```python
from build123d import *

# Parameters (mm, degrees)
SKETCH1_R           = 55
SKETCH1_R_2         = 3
BOSS_EXTRUDE1_DEPTH = 20
SKETCH2_R           = 52
CUT_EXTRUDE1_DEPTH  = 10
SKETCH3_R           = 73.645142789
CUT_EXTRUDE2_DEPTH  = 40
CUT_EXTRUDE4_START  = -58
CUT_EXTRUDE4_DEPTH  = 58
SKETCH5_R           = 2.5
CUT_EXTRUDE3_DEPTH  = 110


with BuildPart() as part:
    # Sketch1 → Boss-Extrude1 (new body)
    with BuildSketch(Plane.XY):
        Circle(SKETCH1_R)
        Circle(SKETCH1_R_2, mode=Mode.SUBTRACT)
    extrude(amount=BOSS_EXTRUDE1_DEPTH)

    # Sketch2 → Cut-Extrude1 (cut)
    with BuildSketch(Plane.XY.offset(20)):
        Circle(SKETCH2_R)
        with BuildLine():
            Line((-41.361950208, 16.620711788), (-41.361950208, -16.620711788))
            ThreePointArc((-41.361950208, -16.620711788), (0, -44.576439802), (41.361950208, -16.620711788))
            Line((41.361950208, -16.620711788), (41.361950208, 16.620711788))
            ThreePointArc((41.361950208, 16.620711788), (0, 44.576439802), (-41.361950208, 16.620711788))
        make_face(mode=Mode.SUBTRACT)
    extrude(amount=-CUT_EXTRUDE1_DEPTH, mode=Mode.SUBTRACT)

    # Sketch3 → Cut-Extrude2 (cut)
    with BuildSketch(Plane.XY.offset(20)):
        Circle(SKETCH3_R)
        with BuildLine():
            Line((-41.361950208, 16.620711788), (-41.361950208, -16.620711788))
            ThreePointArc((-41.361950208, -16.620711788), (0, -44.576439802), (41.361950208, -16.620711788))
            Line((41.361950208, -16.620711788), (41.361950208, 16.620711788))
            ThreePointArc((41.361950208, 16.620711788), (0, 44.576439802), (-41.361950208, 16.620711788))
        make_face(mode=Mode.SUBTRACT)
    extrude(amount=-CUT_EXTRUDE2_DEPTH, mode=Mode.SUBTRACT)

    # Sketch6 → Cut-Extrude4 (cut)
    with BuildSketch(Plane(origin=(0, 0, 0), x_dir=(-1, 0, 0), z_dir=(0, 0, -1)).offset(CUT_EXTRUDE4_START)):
        with BuildLine():
            ThreePointArc((-41.361950208, 16.620711788), (-37.775123844, 23.66641088), (-33, 29.967632295))
            Line((-33, 29.967632295), (-58.675122088, 18.005162572))
            Line((-58.675122088, 18.005162572), (-58.675122088, -19.387832384))
            Line((-58.675122088, -19.387832384), (-33, -29.967632295))
            ThreePointArc((-33, -29.967632295), (-37.775123844, -23.66641088), (-41.361950208, -16.620711788))
            Line((-41.361950208, -16.620711788), (-41.361950208, 16.620711788))
        make_face()
        with BuildLine():
            Line((-33, -29.967632295), (-33, 29.967632295))
            ThreePointArc((-33, 29.967632295), (-37.775123844, 23.66641088), (-41.361950208, 16.620711788))
            Line((-41.361950208, 16.620711788), (-41.361950208, -16.620711788))
            ThreePointArc((-41.361950208, -16.620711788), (-37.775123844, -23.66641088), (-33, -29.967632295))
        make_face()
        with BuildLine():
            Line((59.4434713, 26.815208095), (33, 29.967632295))
            ThreePointArc((33, 29.967632295), (37.775123844, 23.66641088), (41.361950208, 16.620711788))
            Line((41.361950208, 16.620711788), (41.361950208, -16.620711788))
            ThreePointArc((41.361950208, -16.620711788), (37.775123844, -23.66641088), (33, -29.967632295))
            Line((33, -29.967632295), (59.4434713, -14.291474717))
            Line((59.4434713, -14.291474717), (59.4434713, 26.815208095))
        make_face()
        with BuildLine():
            ThreePointArc((41.361950208, 16.620711788), (37.775123844, 23.66641088), (33, 29.967632295))
            Line((33, 29.967632295), (33, -29.967632295))
            ThreePointArc((33, -29.967632295), (37.775123844, -23.66641088), (41.361950208, -16.620711788))
            Line((41.361950208, -16.620711788), (41.361950208, 16.620711788))
        make_face()
    extrude(amount=CUT_EXTRUDE4_DEPTH, mode=Mode.SUBTRACT)

    # Sketch5 → Cut-Extrude3 (cut)
    with BuildSketch(Plane(origin=(33, 0, 0), x_dir=(0, 0, -1), z_dir=(1, 0, 0))):
        with Locations((-8.553262896, -7.517843705)):
            Circle(SKETCH5_R)
        with Locations((-8.553262896, 8.14)):
            Circle(SKETCH5_R)
    extrude(amount=-CUT_EXTRUDE3_DEPTH, mode=Mode.SUBTRACT)


solid = part.part
```
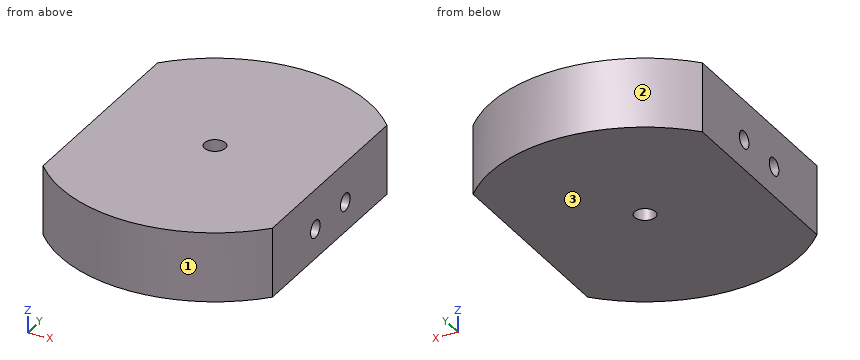
Geometry: final body of the model. Coordinates: model frame, mm. Face numbers are marked on the shaded views. Coordinates: 2 decimals unless noted, no trailing zeros. Order: outer loops, then holes, each group sorted by start corner. A loop starts at its lowest first (then second) coordinate and runs counter-clockwise, first axis right, second up. Notation, with made-up numbers: M 1.5,48 L 42.5,48 A27 cw 42.5,80 Z; hole C 46,21.5 d4. An arc over 180 degrees is marked long. Answer as CSV lines item,"result".
Q1. First-contact query: P1, Ø6.5, axis at y = 8.14, z = 8.55, coming from the +X side; P2, Ø10, axis at x = -20, z = 14, coming from the +Y side; P3, Ø10, axis at x = -20.5, z = 15.5, coming from the -Y side; P4, Ø8, axis at x = 11.5, z = 8.5, coming from the -Y side. Flat tips, straight axial feed; report the tip coordinate or a pass-through.
Answers:
P1,"stops at x = 33"
P2,"stops at y = 41.98"
P3,"stops at y = -41.79"
P4,"stops at y = -43.94"
Q2. Section B-B on x = 0. Return the cut outline in (y, z).
Answers:
outline,"M -44.58,0 L -3,0 L -3,20 L -44.58,20 Z; M 3,0 L 44.58,0 L 44.58,20 L 3,20 Z; hole C -7.52,8.55 d5; hole C 8.14,8.55 d5"
Q3. Section D-D on z = 13.25. Return the cut outline in (x, y), and give its area (3 significant figures).
Answers:
outline,"M -33,-29.97 A44.58 ccw 33,-29.97 L 33,29.97 A44.58 ccw -33,29.97 Z; hole C 0,0 d6"
area,"5,260 mm^2"
Q4. Section A-A on y = 0. Return the cut outline in (x, z), and give its area (3 significant figures).
Answers:
outline,"M -33,0 L -3,0 L -3,20 L -33,20 Z; M 3,0 L 33,0 L 33,20 L 3,20 Z"
area,"1,200 mm^2"
Q5. Section C-C on z = 8.25. Return the cut outline in (x, y), and give its area (3 significant figures).
Answers:
outline,"M -33,-29.97 A44.58 ccw 33,-29.97 L 33,-10 L -33,-10 Z; M -33,-5.04 L 33,-5.04 L 33,5.66 L -33,5.66 Z; M -33,10.62 L 33,10.62 L 33,29.97 A44.58 ccw -33,29.97 Z; hole C 0,0 d6"
area,"4,610 mm^2"
Q6. Line query: probe 1 along Y at (x, z) = (14.5, 9.75); probe 2 along Z at (x, y) = (-13, 8); probe 3 along Y at (x, z) = (-25, 9.25). Output: solid intervals per line, ascending. Write a range as [from, to].
Answers:
probe 1,"y = [-42.15, -9.71], [-5.32, 5.95], [10.33, 42.15]"
probe 2,"z = [0, 6.06], [11.05, 20]"
probe 3,"y = [-36.91, -9.92], [-5.12, 5.74], [10.54, 36.91]"
Q7. Draft query along Y for the marked faces 1, 2 and 3. Return one class per face: pulls with the +Y half, pulls with the -Y half, needs draft (parallel to the pull), parting line crosses it, or undercut.
Answers:
face 1,"pulls with the -Y half"
face 2,"pulls with the +Y half"
face 3,"needs draft"
